Here's how the part is built. I have some questions about the finished solid (model axes, mm). Face numbers are marked on the shaded views. A direction names the side the tool comes from. Coordinates: 2 decimals unless noted, no trailing zeros. Order: outer loops, then holes, each group sorted by start corner. A loop starts at its lowest first (then second) coordinate and runs counter-clockwise, first axis right, second up. Notation, with made-up numbers: M 27,-0.75 L 83,-0.75 A18 cw 83,20.25 Z; hole C 88.25,-10.5 d4. An arc over 180 degrees is marked long. Answer as CSV lines item,"result". Start each with the question number.
Autodesk Fusion 360 part; units mm, degrees
sketch "Sketch1" plane through (0, 0, 0) normal (0, 0, 1) x (1, 0, 0)
  line L0 (20, 19) -> (100, 19)
  line L1 (120, -1) -> (120, -1)
  line L2 (100, -21) -> (20, -21)
  line L3 (0, -1) -> (0, -1)
  line L4 (20.2852, -21) -> (100.2852, -21)
  line L5 (20, 19) -> (100, 19)
  arc A0 (20, 19) -> (0, -1) centre (20, -1) ccw
  arc A1 (0, -1) -> (20, -21) centre (20, -1) ccw
  arc A2 (120, -1) -> (100, 19) centre (100, -1) ccw
  arc A3 (100, -21) -> (120, -1) centre (100, -1) ccw
  circle A4 centre (20, -1.0086) radius 10
  circle A5 centre (100, -1) radius 10
  point P0 (0, 19)
  point P1 (120, 19)
  point P2 (0, -21)
  dimension "d1" = 120
  dimension "d2" = 40
  dimension "d5" = 20
  dimension "d6" = 20
  dimension "d7" = 20
  dimension "d8" = 20
  dimension "d9" = 20
  dimension "d10" = 20
extrude "Extrude1" add sketch "Sketch1" along normal blind 10
sketch "Sketch2" plane through (0, 0, 10) normal (0, 0, 1) x (-1, 0, 0)
  circle A0 centre (-100, 1) radius 10
  circle A1 centre (-20, 1.0086) radius 10
  line L0 (-20, 21) -> (-100, 21)
  arc A2 (-100, 21) -> (-100, -19) centre (-100, 1) ccw
  line L1 (-100, -19) -> (-20, -19)
  arc A3 (-20, -19) -> (-20, 21) centre (-20, 1) ccw
  line L2 (-40, -19) -> (-80, -19)
  line L3 (-80, -19) -> (-80, 21)
  line L4 (-80, 21) -> (-40, 21)
  line L5 (-40, 21) -> (-40, -19)
  dimension "d13" = 40
extrude "Extrude2" add sketch "Sketch2" along normal blind 40 contours L0 L1 L2 L3 L4 L5
fillet "Fillet1" radius 20 2 edges at (40, -1, 50) (80, -1, 50)
sketch "Sketch3" plane through (0, -21, 0) normal (0, -1, 0) x (1, 0, 0)
  arc A0 (80, 30) -> (40, 30) centre (60, 30) ccw
  line L0 (40, 30) -> (40, 10)
  line L1 (40, 10) -> (20, 10)
  line L2 (20, 10) -> (20, 0)
  line L3 (20, 0) -> (100, 0)
  line L4 (100, 0) -> (100, 10)
  line L5 (100, 10) -> (80, 10)
  line L6 (80, 10) -> (80, 30)
  circle A1 centre (60, 30) radius 10
  dimension "d18" = 20
extrude "Extrude3" cut sketch "Sketch3" against normal blind 40 contours A1
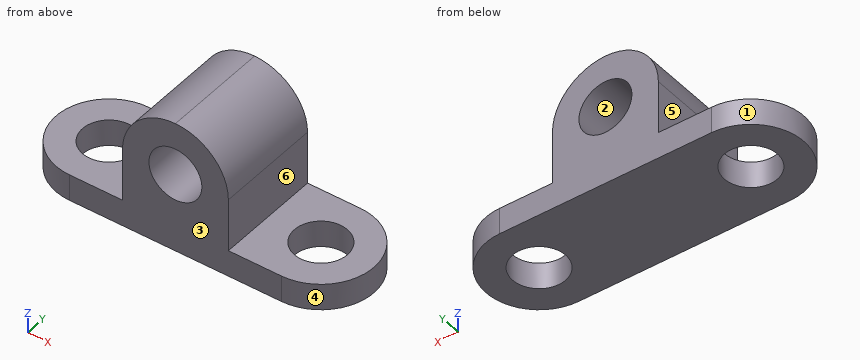
1) I need wall thicknesses on line 1 (Z direction, x = 60, y = -9.5); line 2 (Y direction, x = 20, z = 6); line 3 (X direction, y = -9.5, z = 33). Which ranges of each line are inside material? Lowest first, please. Write a range as [from, to].
2) Will these pins go through, and if not, where does the flat tip stop? pin 1 Ø12 at (x, y) = (94, -1) entering from +Z; pin 2 Ø1.5 at (y, z) = (12, 7.5) entering from +X; pin 3 Ø6 at (y, z) = (1, 19.5) entering from -X.
3) Suppose I cut it at A-A on y = 3. Give the number of separate pieces and of enclosed holes in the cut face, plus the area to 3 significant figures.
4) Suppose I cut it at B-B on z = 32. Please give me the cut outline in (x, y), plus the area to 3 significant figures.
5) Suppose I cut it at D-D on z = 4. Please give me the cut outline in (x, y).
6) If we mould it in two halves opening along X, with no side actions, what happens to the marked faces 1, 2 and 3? For each: released by +X, released by -X, zero draft, split by the parting line, or undercut.
7) Which directions (+Z, -Z, +X, -X, +Y, -Y) give clear straight access to the entire face, cutting with the end or side of a thin tool? Please do the marked faces 4, 5 and 6.
Output:
1,line 1,"[0, 20], [40, 50]"
1,line 2,"[-21, -11.01], [8.99, 19]"
1,line 3,"[40.23, 50.46], [69.54, 79.77]"
2,pin 1,"z = 10"
2,pin 2,"x = 115.81"
2,pin 3,"x = 40"
3,separate pieces,"3"
3,enclosed holes,"1"
3,area,"1,940 mm²"
4,outline,"M 40.1,-21 L 50.2,-21 L 50.2,19 L 40.1,19 Z; M 69.8,-21 L 79.9,-21 L 79.9,19 L 69.8,19 Z"
4,area,"808 mm²"
5,outline,"M 20,-21 L 100,-21 A20 ccw 100,19 L 20,19 A20 ccw Z; hole C 20,-1.01 d20; hole C 100,-1 d20"
6,face 1,"released by -X"
6,face 2,"undercut"
6,face 3,"zero draft"
7,face 4,"+Z, -Z, +X"
7,face 5,"+Z, -X, +Y, -Y"
7,face 6,"+Z, +X, +Y, -Y"
